Part model, mm, in its own coordinate system. Face numbers are marked on the shaded views. A direction names the side the tool comes from. Coordinates: 2 decimals unless noted, no trailing zeros. Order: outer loops, then holes, each group sorted by start corner. A loop starts at its lowest first (then second) coordinate and runs counter-clockwise, first axis right, second up.
1) Mould opens along X. For the marked faces 1, 2, 3 and 4 say: +X half, -X half, draft (parallel to the pull), parting line (faces both ways), or undercut.
2) Tool access for the marked faces 5 and 6: list every direction of +Z, -Z, +X, -X, +Y, -Y with a clear straight run to the whole face (end or side of a thin tool).
3) Wall check: L1, parallel to X at y = 39.5, z = 0.8; L2, parallel to X at y = 9, z = 0.8; L3, parallel to Z at x = 4.15, y = 5. Give the ranges that are in metal, low to high.
4) Cut at C-C (y = 60). List the corners of the cut face in (x, z), and give its area (3 significant figures).
5) Cut at A-A (y = 5). List the corners of the cut face in (x, z).
6) Pin check, flat tips, straight feed: pin 1 Ø0.8 at (x, z) = (5.5, 2) entering from +Y; pin 2 Ø1.5 at (x, z) = (-0.5, 1.5) entering from -Y; pin 3 Ø0.9 at (x, y) = (4.5, 78) entering from -Z. Stop position of each tip, or through.
7) Cut at B-B (x = -3.75). List the corners of the cut face in (y, z), and give its area (3 significant figures).
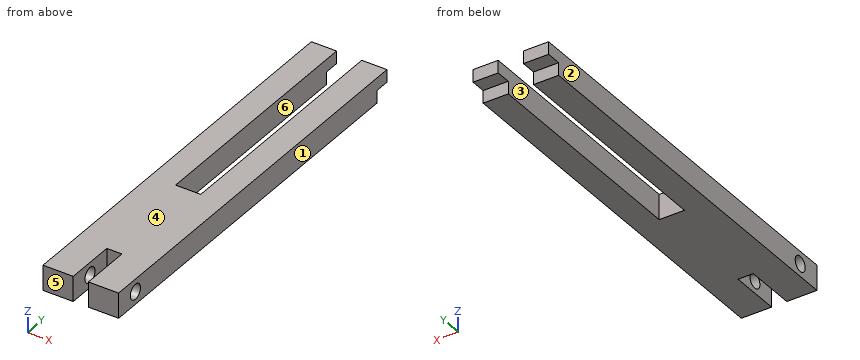
```python
from build123d import *

# Parameters (mm, degrees)
F0_W     = 15
F0_H     = 80
F1_DEPTH = 5
F2_W     = 5
F2_H     = 48
F3_DEPTH = 25
F4_W     = 5
F4_H     = 2.5
F5_DEPTH = 3
F6_W     = 5
F6_H     = 2.5
F7_DEPTH = 3
F8_W     = 3
F8_H     = 10
F9_DEPTH = 25
F11_D    = 3


with BuildPart() as f1:
    # F0 (on Top) → F1 (new body)
    with BuildSketch(Plane.XY):
        with Locations((0, 40)):
            Rectangle(F0_W, F0_H)
    extrude(amount=F1_DEPTH)

    # F2 (on face) → F3 (cut)
    with BuildSketch(Plane.XY.offset(5)):
        with Locations((0, 56)):
            Rectangle(F2_W, F2_H)
    extrude(amount=-F3_DEPTH, mode=Mode.SUBTRACT)

    # F4 (on face) → F5 (cut)
    with BuildSketch(Plane(origin=(0, 80, 0), x_dir=(-1, 0, 0), z_dir=(0, 1, 0))):
        with Locations((5, 1.25)):
            Rectangle(F4_W, F4_H)
    extrude(amount=-F5_DEPTH, mode=Mode.SUBTRACT)

    # F6 (on face) → F7 (cut)
    with BuildSketch(Plane(origin=(0, 80, 0), x_dir=(-1, 0, 0), z_dir=(0, 1, 0))):
        with Locations((-5, 1.25)):
            Rectangle(F6_W, F6_H)
    extrude(amount=-F7_DEPTH, mode=Mode.SUBTRACT)

    # F8 (on face) → F9 (cut)
    with BuildSketch(Plane.XY.offset(5)):
        with Locations((0, 5)):
            Rectangle(F8_W, F8_H)
    extrude(amount=-F9_DEPTH, mode=Mode.SUBTRACT)

    # F11 (through all)
    with Locations(Plane.YZ.offset(7.5)):
        with Locations((5, 2.5)):
            Hole(F11_D / 2)


solid = f1.part
```
Geometry check:
1. face 1: +X half
1. face 2: -X half
1. face 3: undercut
1. face 4: draft
2. face 5: +Z, -Z, +X, -X, -Y
2. face 6: +Z, -Z, +Y
3. L1: x = -7.5 to -2.5, 2.5 to 7.5
3. L2: x = -7.5 to -1.5, 1.5 to 7.5
3. L3: z = 0 to 1, 4 to 5
4. outline: (-7.5, 0) - (-2.5, 0) - (-2.5, 5) - (-7.5, 5) - close; (2.5, 0) - (7.5, 0) - (7.5, 5) - (2.5, 5) - close
4. area: 50.0 mm2
5. outline: (-7.5, 0) - (-1.5, 0) - (-1.5, 1) - (-7.5, 1) - close; (-7.5, 4) - (-1.5, 4) - (-1.5, 5) - (-7.5, 5) - close; (1.5, 0) - (7.5, 0) - (7.5, 1) - (1.5, 1) - close; (1.5, 4) - (7.5, 4) - (7.5, 5) - (1.5, 5) - close
6. pin 1: stops at y = 77
6. pin 2: stops at y = 10
6. pin 3: stops at z = 2.5
7. outline: (0, 0) - (77, 0) - (77, 2.5) - (80, 2.5) - (80, 5) - (0, 5) - close; hole circle Ø3 at (5, 2.5)
7. area: 385 mm2
